Geometry check sheet. Reference: the model listing, model coordinates, mm. A direction names the side the tool comes from. Round coordinates to 2 decimals unless told otherwise and drop trailing zeros. Order: outer loops, then holes, each group sorted by start corner. A loop starts at its lowest first (then second) coordinate and runs counter-clockwise, first axis right, second up. Notation, with made-up numbers: (-29, 87.5) - (-17, 87.5) arc R21 cw to (-17, 120.5) - close; hole circle Ø6 at (17.25, 67.5). An arc over 180 degrees is marked (long way). Write each question's results on one line, items separated by ' | '.
```python
from build123d import *

# Parameters (mm, degrees)
SKETCH1_W                = 457.2
SKETCH1_H                = 190.5
BOSS_EXTRUDE1_DEPTH      = 25.4
SKETCH2_W                = 457.2
SKETCH2_H                = 10.16
BOSS_EXTRUDE2_DEPTH      = 10.16
BOSS_EXTRUDE3_START      = -13.335
SKETCH3_W                = 457.2
SKETCH3_H                = 3.81
BOSS_EXTRUDE3_DEPTH      = 16.51
SKETCH5_W                = 457.2
SKETCH5_H                = 50.8
BOSS_EXTRUDE4_DEPTH      = 19.05
SKETCH6_W                = 441.96
SKETCH6_H                = 20.32
CUT_EXTRUDE1_DEPTH       = 12.7
CUT_EXTRUDE2_DEPTH       = 27.94
CUT_EXTRUDE2_DEPTH_BACK  = 7.62
SKETCH7_W                = 441.96
SKETCH7_H                = 6.35
BOSS_EXTRUDE5_DEPTH      = 25.4
BOSS_EXTRUDE5_DEPTH_BACK = 25.4


with BuildPart() as part:
    # Sketch1 → Boss-Extrude1 (new body)
    with BuildSketch(Plane(origin=(0, 0, 0), x_dir=(1, 0, 0), z_dir=(0, 1, 0))):
        Rectangle(SKETCH1_W, SKETCH1_H)
    extrude(amount=BOSS_EXTRUDE1_DEPTH)

    # Sketch2 → Boss-Extrude2 (add)
    with BuildSketch(Plane.XY.offset(95.25)):
        with Locations((0, 12.7)):
            Rectangle(SKETCH2_W, SKETCH2_H)
    boss_extrude2 = extrude(amount=BOSS_EXTRUDE2_DEPTH)

    # Sketch3 → Boss-Extrude3 (add)
    with BuildSketch(Plane(origin=(0, 17.78, 0), x_dir=(1, 0, 0), z_dir=(0, 1, 0)).offset(BOSS_EXTRUDE3_START)):
        with Locations((0, -103.505)):
            Rectangle(SKETCH3_W, SKETCH3_H)
    boss_extrude3 = extrude(amount=BOSS_EXTRUDE3_DEPTH)

    # Mirror1: Boss-Extrude2, Boss-Extrude3 across plane
    add(boss_extrude2.mirror(Plane.XY))
    add(boss_extrude3.mirror(Plane.XY))

    # Sketch5 → Boss-Extrude4 (add)
    with BuildSketch(Plane(origin=(0, 25.4, 0), x_dir=(1, 0, 0), z_dir=(0, 1, 0))):
        Rectangle(SKETCH5_W, SKETCH5_H)
    extrude(amount=BOSS_EXTRUDE4_DEPTH)

    # Sketch6 → Cut-Extrude1 (cut)
    with BuildSketch(Plane(origin=(0, 44.45, 0), x_dir=(1, 0, 0), z_dir=(0, 1, 0))):
        with Locations((7.62, 0)):
            Rectangle(SKETCH6_W, SKETCH6_H)
    extrude(amount=-CUT_EXTRUDE1_DEPTH, mode=Mode.SUBTRACT)

    # Sketch7 → Cut-Extrude2 (cut, two sides: drawn at the far end of the back side and taken through both)
    with BuildSketch(Plane(origin=(0, 0, 10.16), x_dir=(-1, 0, 0), z_dir=(0, 0, -1)).offset(-CUT_EXTRUDE2_DEPTH_BACK)):
        with Locations((-7.62, 34.925)):
            Rectangle(SKETCH7_W, SKETCH7_H)
    extrude(amount=CUT_EXTRUDE2_DEPTH + CUT_EXTRUDE2_DEPTH_BACK, mode=Mode.SUBTRACT)

    # Sketch8 → Boss-Extrude5 (add, two sides: drawn at the far end of the back side and taken through both)
    with BuildSketch(Plane.XY.offset(-BOSS_EXTRUDE5_DEPTH_BACK)):
        Polygon((44.081942035, 0), (-32.118057965, 0), (-25.4, -38.1), align=None)
    extrude(amount=BOSS_EXTRUDE5_DEPTH + BOSS_EXTRUDE5_DEPTH_BACK)


solid = part.part
```
(1) Section check C-C (y = -16). Record the cut outline in (x, z), then the cut area to 3 significant figures.
Answers follow:
outline: (-29.3, -25.4) - (14.9, -25.4) - (14.9, 25.4) - (-29.3, 25.4) - close | area: 2,250 mm²
(2) Depth check by flat-ended pin: pin 1 Ø8.5 at (x, y) = (-65.5, 23) entering from -Z; pin 2 Ø5 at (x, y) = (24.5, 42) entering from +Z; pin 3 Ø1 at (y, z) = (-7, -4.5) entering from -X; pin 4 Ø4 at (x, z) = (-97.5, -64) entering from -Y. Enter the tip coordinate at first touch or a pass-through.
Answers follow:
pin 1: z = -105.41 | pin 2: z = 25.4 | pin 3: x = -30.97 | pin 4: y = 0
(3) Material ranges on line 1 (Y direction, x = -130, z = 48); line 2 (Z direction, x = 98, y = 26); line 3 (Z direction, x = 91, y = 4), recorded low to high.
Answers follow:
line 1: 0 to 25.4 | line 2: -25.4 to 25.4 | line 3: -95.25 to 95.25
(4) Draft check along Z on faces 1 (the face through (11, 31.75, 0)), 2 (the face through (-3, 25.4, 60)), 3 (the face through (-3, 35, 25.4)). Enter one of: released by +Z, released by -Z, zero draft, split by the parting line, or undercut.
Answers follow:
face 1: undercut | face 2: zero draft | face 3: released by +Z
(5) Section check B-B (z = -50). Record the cut outline in (x, y), then the cut area to 3 significant figures.
Answers follow:
outline: (-228.6, 0) - (228.6, 0) - (228.6, 25.4) - (-228.6, 25.4) - close | area: 11,600 mm²
(6) Access from +Z, -Z, +X, -X, +Y, -Y to the whole of each face (thin tool, end or side, straight path). Record for faces 4 (the face through (-3, -10, 25.4)), 5 (the face through (-3, 35, -25.4)), 6 (the face through (-3, -10, -25.4)), 7 (the face through (-3, 44.45, 11)).
Answers follow:
face 4: +Z, +X, -X, -Y | face 5: -Z, +X, -X, +Y | face 6: -Z, +X, -X, -Y | face 7: +Z, -Z, +X, -X, +Y
